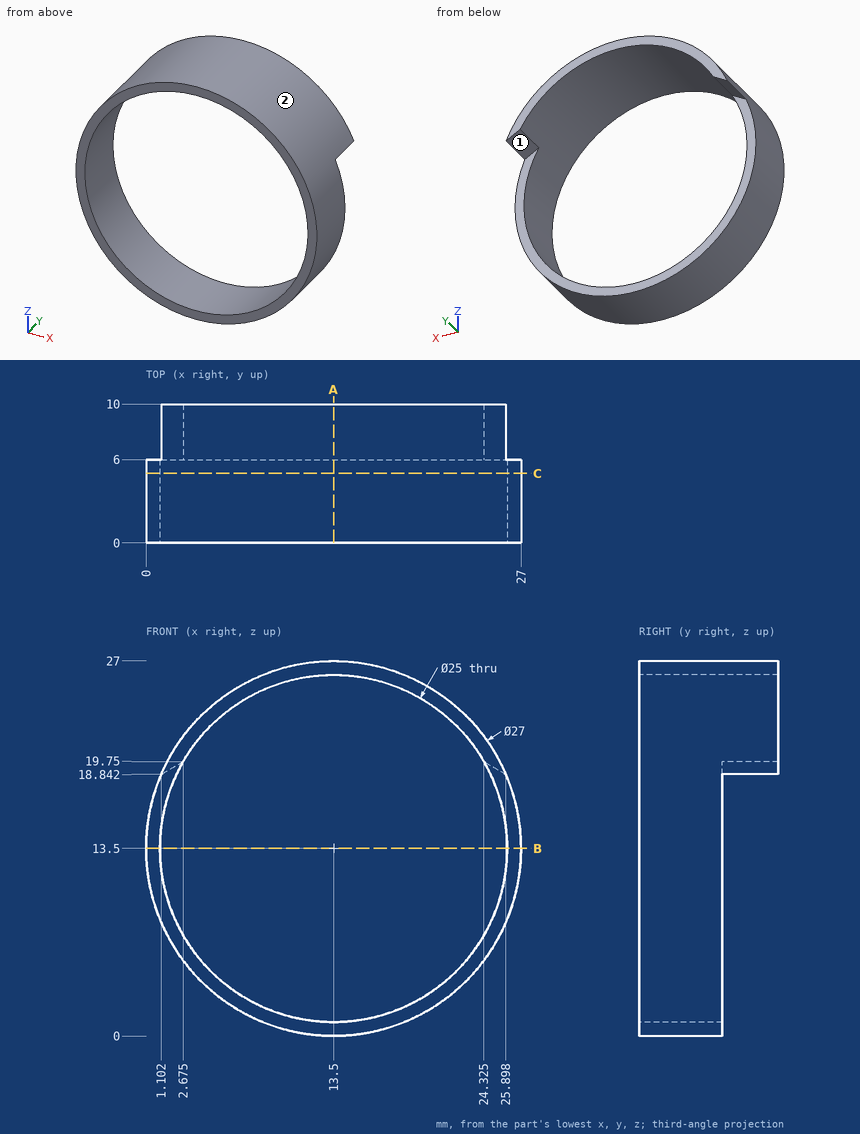
Could you check a few things on this drawing? It's one solid part, dimensions in mm from its lowest x, y, z. Round coordinates to 2 decimals unless told otherwise and drop trailing zeros. Write each loop counter-clockwise with the first axis right and the second up, starting at its lowest first coordinate (ties: lowest second). Pieces come first, ordered by that corner, then holes. Notation, with made-up numbers: M 12.5,-32 L 44.5,-32 A24 cw 44.5,-11 Z; hole C 85.5,-39.5 d6. An arc over 180 degrees is marked long. Answer as CSV lines item,"result". Start each with the question number.
1. Suppose I cut it at C-C on y = 5. Write out the boundary of the cut face in (x, z).
2. Suppose I cut it at A-A on x = 13.5. Write out the boundary of the cut face in (y, z).
3. I need wall thicknesses on probe 1 along X at (y, z) = (2.75, 13.5); probe 2 along Y at (x, z) = (1.5, 8); probe 3 along Z at (x, y) = (21.5, 2.75) (1 decimal). Which ranges of each line are inside material? Lowest first, please.
4. Thinking about a two-plate mould opening in X: for the marked faces 1 and 2, which applies, released by +X, released by -X, zero draft, split by the parting line, or undercut?
5. Suppose I cut it at B-B on z = 13.5. Write out the boundary of the cut face in (x, y), then the cut area to 3 significant figures.
6. I'm going to push flat-ended pins straight in: pin 1 Ø2 at (y, z) = (5.5, 10) entering from +X; pin 2 Ø1.5 at (y, z) = (4, 7.5) entering from +X; pin 3 Ø10 at (x, z) = (5, 6.5) entering from -Y; pin 4 Ø6 at (x, z) = (5, 16.5) entering from +Y. Where does each tip first touch, or does it pass through?
Check result:
1,outline,"C 13.5,13.5 d27; hole C 13.5,13.5 d25"
2,outline,"M 0,0 L 6,0 L 6,1 L 0,1 Z; M 0,26 L 10,26 L 10,27 L 0,27 Z"
3,probe 1,"x = 0 to 1, 26 to 27"
3,probe 2,"y = 0 to 6"
3,probe 3,"z = 2.6 to 3.9, 23.1 to 24.4"
4,face 1,"undercut"
4,face 2,"split by the parting line"
5,outline,"M 0,0 L 1,0 L 1,6 L 0,6 Z; M 26,0 L 27,0 L 27,6 L 26,6 Z"
5,area,"12.0 mm2"
6,pin 1,"stops at x = 26.77"
6,pin 2,"stops at x = 25.94"
6,pin 3,"stops at y = 0"
6,pin 4,"passes through"
